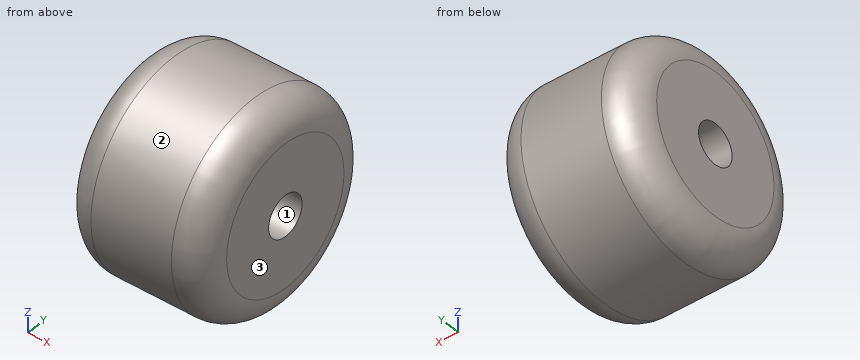
```python
from build123d import *

# Parameters (mm, degrees)
F0_R     = 63.5
F1_DEPTH = 88.9
F2_R     = 19.05
F3_R     = 12.7
F4_DEPTH = 88.901


with BuildPart() as f1:
    # F0 (on Right) → F1 (new body)
    with BuildSketch(Plane.YZ):
        Circle(F0_R)
    extrude(amount=F1_DEPTH)

    # F2
    f2_edges = [f1.edges().sort_by_distance(p)[0] for p in [
        (0, -63.5, 0),
        (44.45, 63.5, 0),
        (88.9, -63.5, 0),
    ]]
    fillet(f2_edges, radius=F2_R)

    # F3 (on face) → F4 (cut, through all)
    with BuildSketch(Plane.YZ.offset(88.9)):
        Circle(F3_R)
    extrude(amount=-F4_DEPTH, mode=Mode.SUBTRACT)


solid = f1.part
```
Build history of the part. All positions in model axes, mm. Face numbers are marked on the shaded views. Coordinates: 2 decimals unless noted, no trailing zeros. Write each loop counter-clockwise with the first axis right and the second up, starting at its lowest first coordinate (ties: lowest second). Pieces come first, ordered by that corner, then holes.
1. Drop flat-ended pins along their axis: pin 1 (8 mm diameter, centred on x = 33, z = 19, fed in from +Y); pin 2 (5 mm diameter, centred on x = 26.5, y = 3.5, fed in from +Z); pin 3 (4 mm diameter, centred on x = 40.5, y = -27.5, fed in from -Z); pin 4 (23 mm diameter, centred on y = 0, z = 0, fed in from -X). Give the stop position or say it passes through.
Answer block:
pin 1: stops at y = 61.7
pin 2: stops at z = 63.49
pin 3: stops at z = -58.15
pin 4: passes through
2. Pull direction Y, two halves, no side cores. Call the marked faces 1, 2 and 3: released by +Y, released by -Y, zero draft, split by the parting line, or undercut.
Answer block:
face 1: undercut
face 2: split by the parting line
face 3: zero draft
3. Drill centre lines: probe 1 along Z at (x, y) = (24, 0); probe 2 along Z at (x, y) = (38, 2.5); probe 3 along Y at (x, z) = (37.5, -39.5). Where is each one in solid material? Low to high.
Answer block:
probe 1: z = -63.5 to -12.7, 12.7 to 63.5
probe 2: z = -63.45 to -12.45, 12.45 to 63.45
probe 3: y = -49.72 to 49.72
4. Band-saw the part on A-A, the plane y = 0. Give the cut face in (x, z), and give its area (3 significant figures).
Answer block:
outline: (0, -44.45) arc R19.05 ccw to (19.05, -63.5) - (69.85, -63.5) arc R19.05 ccw to (88.9, -44.45) - (88.9, -12.7) - (0, -12.7) - close; (0, 12.7) - (88.9, 12.7) - (88.9, 44.45) arc R19.05 ccw to (69.85, 63.5) - (19.05, 63.5) arc R19.05 ccw to (0, 44.45) - close
area: 8,720 mm2
5. Band-saw the part on C-C, the plane x = 32. Give the cut face in (y, z).
Answer block:
outline: circle Ø127 at (0, 0); hole circle Ø25.4 at (0, 0)
